from build123d import *

# Parameters (mm, degrees)
SKETCH_1_W          = 130
SKETCH_1_H          = 100
EXTRUDE_1_DEPTH     = 20
SKETCH_2_W          = 60
SKETCH_2_H          = 76
SKETCH_2_W_2        = 38
CUT_EXTRUDE_1_DEPTH = 10
SKETCH_3_W          = 50
SKETCH_3_H          = 40
EXTRUDE_2_DEPTH     = 65
SKETCH_4_R          = 10
CUT_EXTRUDE_2_DEPTH = 105.642247682
SKETCH_5_R          = 10
CUT_EXTRUDE_3_DEPTH = 121.519707932
SKETCH_6_R          = 10
CUT_EXTRUDE_4_DEPTH = 112.130553854
EXTRUDE_START       = 10
SKETCH_7_W          = 38
SKETCH_7_H          = 76
SKETCH_7_R          = 10
EXTRUDE_3_DEPTH     = 10


with BuildPart() as part:
    # Эскиз1 → Бобышка-Вытянуть1 (new body)
    with BuildSketch(Plane.XY):
        Rectangle(SKETCH_1_W, SKETCH_1_H)
    extrude(amount=EXTRUDE_1_DEPTH)

    # Эскиз2 → Вырез-Вытянуть1 (cut)
    with BuildSketch(Plane.XY.offset(20)):
        with Locations((23, 0)):
            Rectangle(SKETCH_2_W, SKETCH_2_H)
        with Locations((-34, 0)):
            Rectangle(SKETCH_2_W_2, SKETCH_2_H)
    extrude(amount=-CUT_EXTRUDE_1_DEPTH, mode=Mode.SUBTRACT)

    # Эскиз3 → Бобышка-Вытянуть2 (add)
    with BuildSketch(Plane.XY.offset(10)):
        with Locations((40, 30)):
            Rectangle(SKETCH_3_W, SKETCH_3_H)
    extrude(amount=EXTRUDE_2_DEPTH)

    # Эскиз4 → Вырез-Вытянуть2 (cut, through all)
    with BuildSketch(Plane.XY.offset(10)):
        with Locations((-34, 0)):
            Circle(SKETCH_4_R)
    extrude(amount=-CUT_EXTRUDE_2_DEPTH, mode=Mode.SUBTRACT)

    # Эскиз5 → Вырез-Вытянуть3 (cut, through all)
    with BuildSketch(Plane.ZY.offset(-15)):
        with Locations(Location((42.5, 30, 0), (0, 0, 270))):
            Circle(SKETCH_5_R)
    extrude(amount=-CUT_EXTRUDE_3_DEPTH, mode=Mode.SUBTRACT)

    # Эскиз6 → Вырез-Вытянуть4 (cut, through all)
    with BuildSketch(Plane.XY.offset(75)):
        with Locations((40, 30)):
            Circle(SKETCH_6_R)
    extrude(amount=-CUT_EXTRUDE_4_DEPTH, mode=Mode.SUBTRACT)

    # Эскиз7 → Бобышка-Вытянуть3 (add)
    # profile 1 of 2: a face of its own
    with BuildSketch(Plane.XY.offset(10).offset(EXTRUDE_START)):
        Polygon((15, 10), (15, 38), (-7, 38), (-7, -38), (53, -38), (53, 10), align=None)
    # profile 2 of 2: a face of its own
    with BuildSketch(Plane.XY.offset(10).offset(EXTRUDE_START)):
        with Locations((-34, 0)):
            Rectangle(SKETCH_7_W, SKETCH_7_H)
        with Locations((-34, 0)):
            Circle(SKETCH_7_R, mode=Mode.SUBTRACT)
    extrude(amount=-EXTRUDE_3_DEPTH)


solid = part.part
Input: part model. Units: mm. Frame: model coordinates. A direction names the side the tool comes from. Give positions to 0.01 mm unless a question says otherwise; leave off trailing zeros. Order: outer loops, then holes, each group sorted by start corner. A loop starts at its lowest first (then second) coordinate and runs counter-clockwise, first axis right, second up. Notation, with made-up numbers: (67, 59) - (88, 59) arc R17 cw to (88, 77) - close; hole circle Ø2 at (-8, 46.25). An arc over 180 degrees is marked (long way). Write each question's results on one line, items separated by ' | '.
Item 1: Section B-B (x = -34). Return loops of the section in (y, z).
A:
outline: (-50, 0) - (-10, 0) - (-10, 20) - (-50, 20) - close; (10, 0) - (50, 0) - (50, 20) - (10, 20) - close
Item 2: Section C-C (y = 30). Return loops of the section in (x, z).
A:
outline: (-65, 0) - (30, 0) - (30, 32.5) - (15, 32.5) - (15, 20) - (-65, 20) - close; (15, 52.5) - (30, 52.5) - (30, 75) - (15, 75) - close; (50, 0) - (65, 0) - (65, 32.5) - (50, 32.5) - close; (50, 52.5) - (65, 52.5) - (65, 75) - (50, 75) - close
Item 3: Draft query along Y for faces 1 (the cylindrical face through (45.38, 38.43, 16.83)), 2 (the flat face through (40, 10, 47)), 3 (the flat face through (-15, 1, 20)), 4 (the flat face through (28, 50, 29)). Return one class per face: released by +Y, released by -Y, zero draft, split by the parting line, or undercut.
A:
face 1: undercut | face 2: released by -Y | face 3: zero draft | face 4: released by +Y
Item 4: Section A-A (y = 0). Return loops of the section in (x, z).
A:
outline: (-65, 0) - (-44, 0) - (-44, 20) - (-65, 20) - close; (-24, 0) - (65, 0) - (65, 20) - (-24, 20) - close
Item 5: Access query for faces 5 (the flat face through (15, 30, 53)), 6 (the cylindrical face through (24.55, 37.94, 36.42)). Directions: +Z, -Z, +X, -X, +Y, -Y. A direction counts if a zero-diameter tool reaches every point of the face in a straight line with its end or side. Return the directions, or none.
A:
face 5: +Z, -X, +Y, -Y | face 6: +X, -X
Item 6: Section D-D (z = 60.5). Return loops of the section in (x, y).
A:
outline: (15, 10) - (65, 10) - (65, 50) - (15, 50) - close; hole circle Ø20 at (40, 30)
Item 7: Contact query for flat-ended pins moving along their axis: pin 1 Ø4 at (x, z) = (18, 28.5) entering from -Y; pin 2 Ø2 at (x, y) = (25, -17) entering from +Z. Output: stop coordinate, or through.
A:
pin 1: stops at y = 10 | pin 2: stops at z = 20
Item 8: Material intervals for line 1 along Y through (x, z) = (20, 42); line 2 along X through (y, z) = (30, 14.5); line 3 along Z through (x, y) = (22, 30), sorted ascending.
A:
line 1: y = 10 to 20.01, 39.99 to 50 | line 2: x = -65 to 30, 50 to 65 | line 3: z = 0 to 32.5, 52.5 to 75
